from build123d import *

# Parameters (mm, degrees)
SKETCH_1_W          = 19
SKETCH_1_H          = 29
SKETCH_1_W_2        = 20
EXTRUDE_1_DEPTH     = 6
SKETCH_3_R          = 1.5
CUT_EXTRUDE_1_DEPTH = 10
FILLET_1_R          = 3
FILLET_2_R          = 1
SKETCH_4_R          = 1.5
CUT_EXTRUDE_2_DEPTH = 72
FILLET_3_R          = 0.5
FILLET_4_R          = 0.5
FILLET_5_R          = 3
FILLET_6_R          = 2


with BuildPart() as part:
    # 草图1 → 凸台-拉伸1 (new body)
    with BuildSketch(Plane(origin=(0, 0, 0), x_dir=(1, 0, 0), z_dir=(0, 1, 0))):
        with BuildLine():
            Line((17, 0), (50, 0))
            Line((50, 0), (50, 8))
            Line((50, 8), (52.5, 8))
            Line((52.5, 8), (52.5, -3.83484861))
            ThreePointArc((52.5, -3.83484861), (55, -22.5), (57.5, -3.83484861))
            Line((57.5, -3.83484861), (57.5, 8))
            Line((57.5, 8), (60, 8))
            Line((60, 8), (60, -2.091287885))
            ThreePointArc((60, -2.091287885), (65.099504938, -6.519259302), (67, -13))
            Line((67, -13), (67, -22.5))
            Line((67, -22.5), (68, -22.5))
            Line((68, -22.5), (68, -57))
            Line((68, -57), (0, -57))
            Line((0, -57), (0, -13))
            ThreePointArc((0, -13), (1.900495062, -6.519259302), (7, -2.091287885))
            Line((7, -2.091287885), (7, 8))
            Line((7, 8), (9.5, 8))
            Line((9.5, 8), (9.5, -3.83484861))
            ThreePointArc((9.5, -3.83484861), (12, -22.5), (14.5, -3.83484861))
            Line((14.5, -3.83484861), (14.5, 8))
            Line((14.5, 8), (17, 8))
            Line((17, 8), (17, 0))
        make_face()
        with Locations((12.5, -39.5)):
            Rectangle(SKETCH_1_W, SKETCH_1_H, mode=Mode.SUBTRACT)
        Polygon((24, -25), (24, -54), (43, -54), (43, -25), (43, -4), (24, -4), align=None, mode=Mode.SUBTRACT)
        with Locations((55, -39.5)):
            Rectangle(SKETCH_1_W_2, SKETCH_1_H, mode=Mode.SUBTRACT)
    extrude(amount=EXTRUDE_1_DEPTH)

    # 草图3 → 切除-拉伸1 (cut)
    with BuildSketch(Plane.XY.offset(57)):
        with Locations((12, 3)):
            Circle(SKETCH_3_R)
        with Locations((32, 3)):
            Circle(SKETCH_3_R)
        with Locations((52, 3)):
            Circle(SKETCH_3_R)
    extrude(amount=-CUT_EXTRUDE_1_DEPTH, mode=Mode.SUBTRACT)

    # 圆角1
    fillet_1_edges = [part.edges().sort_by_distance(p)[0] for p in [
        (22, 3, 25),
        (3, 3, 25),
        (3, 3, 54),
        (22, 3, 54),
        (24, 3, 4),
        (24, 3, 54),
        (43, 3, 54),
        (43, 3, 4),
        (45, 3, 54),
        (65, 3, 54),
        (65, 3, 25),
        (45, 3, 25),
    ]]
    fillet(fillet_1_edges, radius=FILLET_1_R)

    # 圆角2
    fillet_2_edges = [part.edges().sort_by_distance(p)[0] for p in [
        (50, 3, 0),
        (17, 3, 0),
        (68, 3, 22.5),
    ]]
    fillet(fillet_2_edges, radius=FILLET_2_R - 0.0001)  # a hair under: the kernel refuses the full size

    # 草图4 → 切除-拉伸2 (cut)
    with BuildSketch(Plane.ZY.offset(-7)):
        with Locations((-4, 3)):
            Circle(SKETCH_4_R)
    extrude(amount=-CUT_EXTRUDE_2_DEPTH, mode=Mode.SUBTRACT)

    # 圆角3
    fillet_3_edges = [part.edges().sort_by_distance(p)[0] for p in [
        (68, 3, 57),
        (0, 3, 57),
    ]]
    fillet(fillet_3_edges, radius=FILLET_3_R)

    # 圆角4
    fillet_4_edges = [part.edges().sort_by_distance(p)[0] for p in [
        (7, 3, -8),
        (17, 3, -8),
        (50, 3, -8),
        (60, 3, -8),
    ]]
    fillet(fillet_4_edges, radius=FILLET_4_R)

    # 圆角5
    fillet_5_edges = [part.edges().sort_by_distance(p)[0] for p in [
        (7, 3, 2.091287885),
        (60, 3, 2.091287885),
    ]]
    fillet(fillet_5_edges, radius=FILLET_5_R)

    # 圆角6
    fillet_6_edges = [part.edges().sort_by_distance(p)[0] for p in [
        (9.5, 3, 3.83484861),
        (14.5, 3, 3.83484861),
        (52.5, 3, 3.83484861),
        (57.5, 3, 3.83484861),
    ]]
    fillet(fillet_6_edges, radius=FILLET_6_R)


solid = part.part
Source: CAD feature listing. Evaluate the final solid. Frame: model axes, mm. A direction names the side the tool comes from. Give positions to 0.01 mm unless a question says otherwise; leave off trailing zeros. Write each loop counter-clockwise with the first axis right and the second up, starting at its lowest first coordinate (ties: lowest second). Pieces come first, ordered by that corner, then holes. Notation, with made-up numbers: M 36.25,5 L 63.25,5 A15 cw 63.25,33 Z; hole C 69.25,11.25 d3. An arc over 180 degrees is marked long. Return JSON: item names as keys, results as strings. Group by question number.
1) Set-up query: faces 1 (the face through (57.823, 3.042, 3.507)), 2 (the face through (67, 3, 18)), 3 (the face through (15.73, 1.67, -3.31)), 4 (the face through (57.5, 3, -2)), 5 (the face through (30.5, 3.07, 55.52)). Return all of +Z, -Z, +X, -X, +Y, -Y with unobstructed straight access to the full face (end or side cutting, diameter ignored); none if empty.
2) Cut plane A-A, the plane z = -4. Give the number of separate pieces and of enclosed holes in the cut face, plus the area to 3 significant figures.
3) Material intervals for line 1 along X through (y, z) = (3, 42.5); line 2 along X through (y, z) = (5.6, -2.5); line 3 along Y through (x, z) = (51.7, -4), sorted ascending. Write a range as [from, to].
4) Cut plane C-C, the plane x = 55. Output: boundary loops of the cut face in (y, z).
5) Pull-direction query (Y, two-part tool) for faces 6 (the face through (8.23, 1.67, -3.31)), 7 (the face through (22, 3, 40)), 8 (the face through (51.23, 1.67, -3.31)); classes: pulls with the +Y half, pulls with the -Y half, needs draft (parallel to the pull), parting line crosses it, or undercut.
6) Cut plane D-D, the plane z = 39.5. Output: boundary loops of the cut face in (x, y).
7) Cut plane B-B, the plane x = 12. Output: boundary loops of the cut face in (y, z), plus the area to 3 significant figures.
8) Pin query (flat end, axial travel): P1, Ø1.8, axis at x = 52, y = 3, coming from the +Z side; P2, Ø3, axis at y = 2.5, z = 7.5, coming from the +X side. Return the tip coordinate at first contact, or that it passes through.
Recorded:
{
 "1": {"face 1": "+Y, -Y", "face 2": "-Z, +X, +Y, -Y", "face 3": "+X, -X", "face 4": "-Z, +Y, -Y", "face 5": "+Z"},
 "2": {"separate pieces": "8", "enclosed holes": "0", "area": "30.0 mm²"},
 "3": {"line 1": "x = [0, 3], [22, 24], [43, 45], [65, 68]", "line 2": "x = [7, 9.5], [14.5, 17], [50, 52.5], [57.5, 60]", "line 3": "y = [0, 1.5], [4.5, 6]"},
 "4": {"outline": "M 0,22.5 L 6,22.5 L 6,25 L 0,25 Z; M 0,54 L 6,54 L 6,57 L 0,57 Z"},
 "5": {"face 6": "undercut", "face 7": "needs draft", "face 8": "undercut"},
 "6": {"outline": "M 0,0 L 3,0 L 3,6 L 0,6 Z; M 22,0 L 24,0 L 24,6 L 22,6 Z; M 43,0 L 45,0 L 45,6 L 43,6 Z; M 65,0 L 68,0 L 68,6 L 65,6 Z"},
 "7": {"outline": "M 0,22.5 L 6,22.5 L 6,25 L 0,25 Z; M 0,54 L 1.5,54 L 1.5,57 L 0,57 Z; M 4.5,54 L 6,54 L 6,57 L 4.5,57 Z", "area": "24.0 mm²"},
 "8": {"P1": "stops at z = 25", "P2": "stops at x = 66.31"}
}
